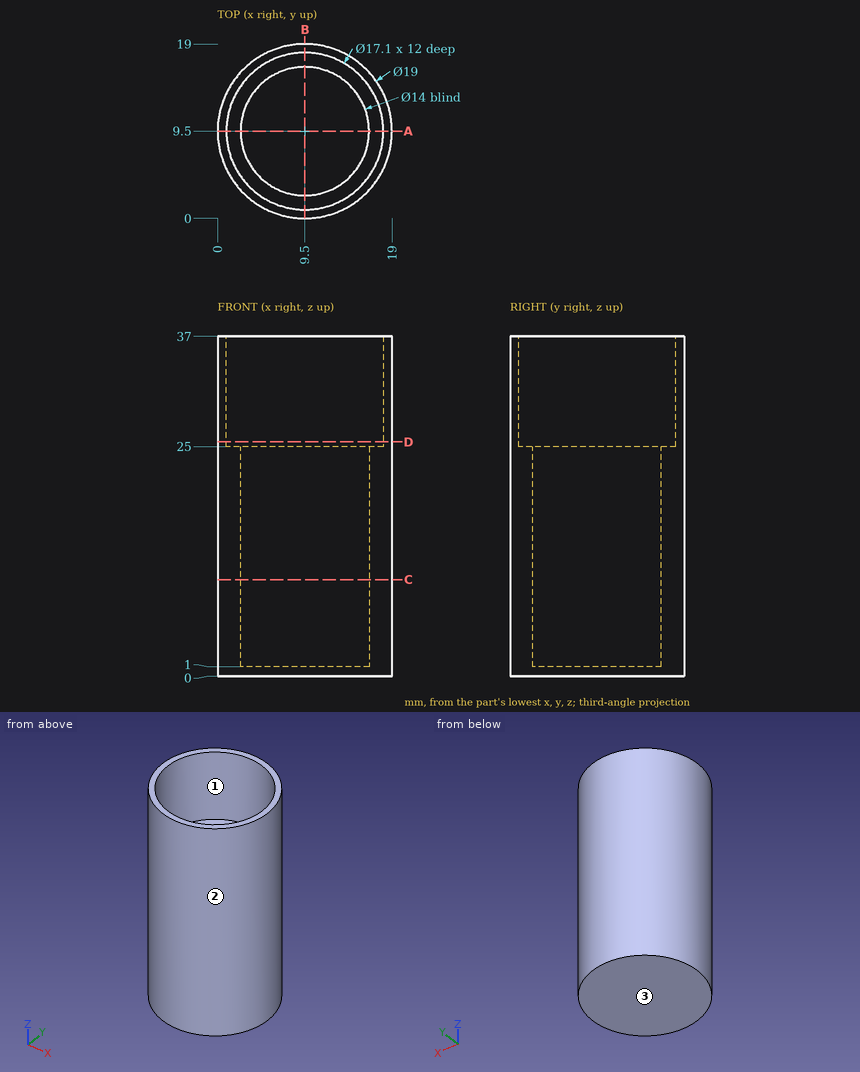
Geometry check sheet. Reference: drawing and pictorial views, mm from the part's lowest x, y, z. Give positions to 0.01 mm unless a question says otherwise; leave off trailing zeros. Loops run counter-clockwise (first coordinate to the right, second up) from the corner with the lowest first, then second, coordinate; pieces in that order, holes last.
1. Section check C-C, the plane z = 10.5. Enter the section's corners in (x, y).
2. Go/stop test with flat-tipped pins: pin 1 Ø5 at (y, z) = (2, 27) entering from -X; pin 2 Ø4 at (y, z) = (15.5, 12) entering from +X; pin 3 Ø5 at (y, z) = (14.5, 31) entering from -X. Record where each tip stops, or that it passes through.
3. Thickness scan on line 1 (Y direction, x = 9.5, z = 31); line 2 (Y direction, x = 9.5, z = 19.25). Record the ranges inside material, lowest first.
4. Section check D-D, the plane z = 25.5. Enter the section's corners in (x, y), then the cut area to 3 significant figures.
5. Section check A-A, the plane y = 9.5. Enter the section's corners in (x, z).
6. Mould release check, pull along Y, two halves, no side actions. Record for the marked faces 1, 2 and 3: released by +Y, released by -Y, zero draft, split by the parting line, or undercut.
Geometry says:
1. outline: circle Ø19 at (9.5, 9.5); hole circle Ø14 at (9.5, 9.5)
2. pin 1: stops at x = 1.42
2. pin 2: stops at x = 18.12
2. pin 3: stops at x = 0.33
3. line 1: y = 0 to 0.95, 18.05 to 19
3. line 2: y = 0 to 2.5, 16.5 to 19
4. outline: circle Ø19 at (9.5, 9.5); hole circle Ø17.1 at (9.5, 9.5)
4. area: 53.9 mm2
5. outline: (0, 0) - (19, 0) - (19, 37) - (18.05, 37) - (18.05, 25) - (16.5, 25) - (16.5, 1) - (2.5, 1) - (2.5, 25) - (0.95, 25) - (0.95, 37) - (0, 37) - close
6. face 1: undercut
6. face 2: split by the parting line
6. face 3: zero draft
